Source: CAD feature listing. Evaluate the final solid. Frame: model axes, mm. A direction names the side the tool comes from. Coordinates: 2 decimals unless noted, no trailing zeros. Order: outer loops, then holes, each group sorted by start corner. A loop starts at its lowest first (then second) coordinate and runs counter-clockwise, first axis right, second up.
```python
from build123d import *

# Parameters (mm, degrees)
F1_DEPTH = 4
F2_R     = 1
F3_DEPTH = 11
F5_DEPTH = 15
F6_R     = 0.99999
F7_R     = 0.4


# Not quite as in the source:
# - a fillet or chamfer that OpenCascade refuses, or shapes differently, is made with other operations: its cross-section is extruded or revolved along the edge and cut away or added
# - a fillet or chamfer is up to 0.001 mm smaller than in the source, because OpenCascade refuses the exact size
# - a feature names something its author has since deleted; it is built from what else it names


with BuildPart() as f1:
    # F0 (on Top) → F1 (new body)
    with BuildSketch(Plane.XY):
        with BuildLine():
            ThreePointArc((-4.75, -2.7726341266), (-1.4361406616, 5.3091901454), (5.5, 0))
            ThreePointArc((5.5, 0), (5.3091901454, -1.4361406616), (4.75, -2.7726341266))
            Line((4.75, -2.7726341266), (6.9686799324, -2.7726341266))
            ThreePointArc((6.9686799324, -2.7726341266), (7.3659724237, -1.4115418001), (7.5, 0))
            ThreePointArc((7.5, 0), (5.3033008589, 5.3033008589), (0, 7.5))
            ThreePointArc((0, 7.5), (-5.3033008589, 5.3033008589), (-7.5, 0))
            ThreePointArc((-7.5, 0), (-7.3659724237, -1.4115418001), (-6.9686799324, -2.7726341266))
            Line((-6.9686799324, -2.7726341266), (-4.75, -2.7726341266))
        make_face()
        with BuildLine():
            ThreePointArc((0, 7.5), (5.3033008589, 5.3033008589), (7.5, 0))
            Line((7.5, 0), (7.5, 7.5))
            Line((7.5, 7.5), (0, 7.5))
        make_face()
    extrude(amount=F1_DEPTH)

    # F2 (on face) → F3 (join)
    with BuildSketch(Plane.XY.offset(4)):
        with Locations((0, 6.5)):
            Circle(F2_R)
        with BuildLine():
            ThreePointArc((0, 7.5), (0.7071067812, 7.2071067812), (1, 6.5))
            ThreePointArc((1, 6.5), (0.7071067812, 5.7928932188), (0, 5.5))
            ThreePointArc((0, 5.5), (4.769669155, 2.7386595538), (4.75, -2.7726341266))
            Line((4.75, -2.7726341266), (6.9686799324, -2.7726341266))
            ThreePointArc((6.9686799324, -2.7726341266), (7.3659724237, -1.4115418001), (7.5, 0))
            Line((7.5, 0), (7.5, 7.5))
            Line((7.5, 7.5), (0, 7.5))
        make_face()
    extrude(amount=F3_DEPTH)

    # F4 (on face) → F5 (join, through all)
    with BuildSketch(Plane.XY.offset(15)):
        with BuildLine():
            Line((7.5, 6.25), (7.5, 2.65))
            Line((7.5, 2.65), (7.5, 0))
            ThreePointArc((7.5, 0), (7.4864300086, -0.4509608915), (7.4457691398, -0.9002899069))
            ThreePointArc((7.4457691398, -0.9002899069), (10.1065360675, -2.1571253539), (13.0041807725, -1.6443182282))
            ThreePointArc((13.0041807725, -1.6443182282), (14.900619035, 0.1410437177), (15.6, 2.65))
            ThreePointArc((15.6, 2.65), (14.1794678888, 6.0794678888), (10.75, 7.5))
            ThreePointArc((10.75, 7.5), (9.0089514654, 7.1767261901), (7.5, 6.25))
        make_face()
        with BuildLine():
            ThreePointArc((7.5, 2.65), (10.75, 5.9), (14, 2.65))
            ThreePointArc((14, 2.65), (10.75, -0.6), (7.5, 2.65))
        make_face(mode=Mode.SUBTRACT)
        with BuildLine():
            Line((7.5, 0), (7.5, 2.65))
            Line((7.5, 2.65), (7.5, 6.25))
            ThreePointArc((7.5, 6.25), (6.712321746, 5.3369414428), (6.1742445242, 4.2577816473))
            ThreePointArc((6.1742445242, 4.2577816473), (7.1608949836, 2.2297046967), (7.5, 0))
        make_face()
        with BuildLine():
            ThreePointArc((7.4457691398, -0.9002899069), (7.4864300086, -0.4509608915), (7.5, 0))
            ThreePointArc((7.5, 0), (7.1608949836, 2.2297046967), (6.1742445242, 4.2577816473))
            ThreePointArc((6.1742445242, 4.2577816473), (6.0409691333, 1.4891691352), (7.4457691398, -0.9002899069))
        make_face()
        with BuildLine():
            Line((7.5, 7.5), (7.5, 6.25))
            ThreePointArc((7.5, 6.25), (9.0089514654, 7.1767261901), (10.75, 7.5))
            Line((10.75, 7.5), (7.5, 7.5))
        make_face()
        with BuildLine():
            ThreePointArc((13.0041807725, -1.6443182282), (10.1065360675, -2.1571253539), (7.4457691398, -0.9002899069))
            ThreePointArc((7.4457691398, -0.9002899069), (7.2677715796, -1.8518899176), (6.9686799324, -2.7726341266))
            ThreePointArc((6.9686799324, -2.7726341266), (5.5735770486, -5.0184897015), (3.4858465555, -6.640698291))
            Line((3.4858465555, -6.640698291), (13.0041807725, -1.6443182282))
        make_face()
        with BuildLine():
            ThreePointArc((3.4858465555, -6.640698291), (5.5735770486, -5.0184897015), (6.9686799324, -2.7726341266))
            Line((6.9686799324, -2.7726341266), (4.75, -2.7726341266))
            ThreePointArc((4.75, -2.7726341266), (2.7386595462, -4.7696691594), (-1.76e-08, -5.5))
            ThreePointArc((-1.76e-08, -5.5), (0.707106775, -5.7928932126), (1, -6.5))
            ThreePointArc((1, -6.5), (0.7071067812, -7.2071067812), (0, -7.5))
            ThreePointArc((0, -7.5), (1.7950992755, -7.2820064949), (3.4858465555, -6.640698291))
        make_face()
        with BuildLine():
            ThreePointArc((-1.76e-08, -5.5), (-1, -6.5000000088), (0, -7.5))
            ThreePointArc((0, -7.5), (0.7071067812, -7.2071067812), (1, -6.5))
            ThreePointArc((1, -6.5), (0.707106775, -5.7928932126), (-1.76e-08, -5.5))
        make_face()
    extrude(amount=-F5_DEPTH)

    # F6 (radius 1 in the source; OpenCascade refuses exactly that, so slightly less here)
    f6_edges = [f1.edges().sort_by_distance(p)[0] for p in [
        (-6.96868, -2.772634, 2),
        (-4.75, -2.772634, 2),
    ]]
    fillet(f6_edges, radius=F6_R)

    # F7
    f7_edges = [f1.edges().sort_by_distance(p)[0] for p in [
        (8.245014, -4.142508, 15),
        (3.75, 7.5, 15),
        (4.769669, 2.73866, 15),
        (-1, 6.5, 15),
        (9.125, 7.5, 15),
        (15.459031, 3.810831, 15),
        (1.795099, -7.282006, 15),
        (-1, -6.5, 15),
        (2.73866, -4.769669, 15),
    ]]
    fillet(f7_edges, radius=F7_R)

    # F8: chamfer of 1 on 1 edges, made by hand

    # F8_s1 → F8_t2 (revolve, cut)
    with BuildSketch(Plane.XZ.offset(-2.65)):
        Polygon((6.5, 0), (7.5, 1), (7.5, 0), align=None)
    revolve(axis=Axis((10.75, 2.65, 0), (0, 0, -1)), mode=Mode.SUBTRACT)

    # F9: fillet of radius 20 on 1 edges, made by hand

    # F9_s1 → F9_t2 (revolve, cut)
    with BuildSketch(Plane.XZ.offset(-2.65)):
        with BuildLine():
            ThreePointArc((7.5, 6.2449979984), (7.2484176581, 3.0827203382), (6.5, 0))
            Line((6.5, 0), (7.5, 1))
            Line((7.5, 1), (7.5, 6.2449979984))
        make_face()
    revolve(axis=Axis((10.75, 2.65, 1), (0, 0, -1)), mode=Mode.SUBTRACT)


solid = f1.part
```
1. Draft query along Y for faces 1 (the cylindrical face through (-1, -6.5, 7.4)), 2 (the flat face through (7, 2, 15)), 3 (the cylindrical face through (8.259, -4.007, 14.88)). Return one class per face: +Y half, -Y half, draft (parallel to the pull), parting line (faces both ways), or undercut.
2. Section query D-D, the plane z = 4.75. Output: boundary loops of the cut face in (x, y).
3. Section query A-A, the plane z = 10.5. Output: boundary loops of the cut face in (x, y), plus the area to 3 significant figures.
4. Section query C-C, the plane x = -3.25. Output: boundary loops of the cut face in (y, z), plus the area to 3 significant figures.
5. Access query for faces 4 (the flat face through (5, 3, 0)), 5 (the cylindrical face through (-1, 6.5, 9.2)). Directions: +Z, -Z, +X, -X, +Y, -Y. A direction counts if a zero-diameter tool reaches every point of the face in a straight line with its end or side. Return the directions, or none.
6. Material intervals for line 1 along X through (y, z) = (1, 1.25); line 2 along Y through (x, z) = (0, 1.6); line 3 along X through (y, z) = (4.5, 2.25), sorted ascending.
7. Contact query for flat-ended pins moving along their axis: P1, Ø6, axis at y = -3, z = 11, coming from the -X side; P2, Ø6, axis at y = 6, z = 8.5, coming from the +X side; P3, Ø4, axis at x = 12, z = 9, coming from the -Y side. Output: stop coordinate, or through.
Answer key:
1. face 1: undercut
1. face 2: draft
1. face 3: -Y half
2. outline: (0, -7.5) arc R7.5 ccw to (3.49, -6.64) - (13, -1.64) arc R4.85 ccw to (10.75, 7.5) - (0, 7.5) arc R1 ccw to (0, 5.5) arc R5.5 cw to (0, -5.5) arc R1 ccw to start; hole circle Ø6.61 at (10.75, 2.65)
3. outline: (0, -7.5) arc R7.5 ccw to (3.49, -6.64) - (13, -1.64) arc R4.85 ccw to (10.75, 7.5) - (0, 7.5) arc R1 ccw to (0, 5.5) arc R5.5 cw to (0, -5.5) arc R1 ccw to start; hole circle Ø6.5 at (10.75, 2.65)
3. area: 100 mm2
4. outline: (4.44, 0) - (6.76, 0) - (6.76, 4) - (4.44, 4) - close
4. area: 9.29 mm2
5. face 4: -Z, +X, -X, +Y, -Y
5. face 5: +Z, -X
6. line 1: x = -7.43 to -5.41, 5.41 to 7.23, 14.27 to 15.31
6. line 2: y = -7.5 to -5.5, 5.5 to 7.5
6. line 3: x = -6 to -3.16, 3.16 to 7.6, 13.9 to 15.23
7. P1: stops at x = -0.87
7. P2: stops at x = 15.59
7. P3: stops at y = -3.22
